Verification items for the finished model (mm, model axes). A direction names the side the tool comes from. Coordinates: 2 decimals unless noted, no trailing zeros. Loops run counter-clockwise (first coordinate to the right, second up) from the corner with the lowest first, then second, coordinate; pieces in that order, holes last. Notation, with made-up numbers: (-19, -22.5) - (-11, -22.5) arc R17 ccw to (-11, -7.5) - close; hole circle Ø7 at (-29.75, 40). An arc over 180 degrees is marked (long way). One line per item, written item: value. Start each with the question number.
(1) Section check A-A (y = 0). Record the boundary of the cut face in (x, z).
(2) Thickness scan on probe 1 along X at (y, z) = (101, -55); probe 2 along X at (y, z) = (-50, 64); probe 3 along Z at (x, y) = (117, -12). Record the ranges inside material, lowest first. Write a range as [from, to].
(3) Section check C-C (x = -96). Record the boundary of the cut face in (y, z).
(4) Section check B-B (z = -59). Count the separate pieces of the cut face and the enclosed holes in it, plus the area to 3 significant figures.
(5) Set-up check for faces 1 (the face through (-35.487, 74.751, 18.458)), 2 (the face through (-153.15, 71.8, -13.56)), 3 (the face through (-75, 99, 1)), 4 (the face through (62.59, 99.15, 59.84)): record each of +Z, -Z, +X, -X, +Y, -Y from which the full face is reachable in a straight line by a thin tool's end or side.
(6) Gauge pin test, flat ends, axial feed: P1, Ø16, axis at x = -55, z = 55, coming from the -Y side; P2, Ø1, axis at x = -121, y = 8, coming from the -Z side; P3, Ø6.5, axis at x = 25.5, y = 103, coming from the +Z side; P4, Ø23.5, axis at y = -20.71, z = 77.27, coming from the -X side. Record the tip position at first contact, or that the pin passes through.
(7) Draft check along X on faces 5 (the face through (-69.297, 99.154, -68.986)), 6 (the face through (-142, 43, -43)), 7 (the face through (153.15, 56.96, 65.56)). Enter one of: +X half, -X half, draft (parallel to the pull), parting line (faces both ways), or undercut.
```python
from build123d import *

# Parameters (mm, degrees)
SKETCH2_R           = 40
SKETCH2_R_2         = 9
BOSS_EXTRUDE1_DEPTH = 22
BOSS_EXTRUDE6_REACH = 286.598
SKETCH2_8_R         = 40
SKETCH2_8_R_2       = 27.5
SKETCH2_8_R_3       = 24
CUT_EXTRUDE5_REACH  = 362.117
SKETCH8_R           = 9


with BuildPart() as part:
    # Sketch1 → Revolve1 (revolve)
    with BuildSketch(Plane.XY, mode=Mode.PRIVATE) as revolve1_sk:
        Polygon((-164, -37.5), (-164, -100), (-142, -100), (-142, -54.482048161), (0, -66.905438381), (142, -54.482048161), (142, -100), (164, -100), (164, -37.5), (0, -51.848140818), align=None)
    revolve(revolve1_sk.sketch.rotate(Axis((0, 0, 0), (-1, 0, 0)), 270), axis=Axis((0, 0, 0), (-1, 0, 0)))

    # Sketch2<8> → Boss-Extrude6 (add, up to next)
    with BuildSketch(Plane(origin=(0, 110, 0), x_dir=(1, 0, 0), z_dir=(0, 1, 0)), mode=Mode.PRIVATE) as boss_extrude6_sk1:
        with Locations(Location((0, 0, 0), (0, 0, 270))):
            Circle(SKETCH2_8_R)
        Circle(SKETCH2_8_R_2, mode=Mode.SUBTRACT)
    boss_extrude6_tool1 = extrude(boss_extrude6_sk1.sketch, amount=-BOSS_EXTRUDE6_REACH, mode=Mode.PRIVATE) - part.part
    # Sketch2<8> → Boss-Extrude6 (add, up to next)
    with BuildSketch(Plane(origin=(0, 110, 0), x_dir=(1, 0, 0), z_dir=(0, 1, 0)), mode=Mode.PRIVATE) as boss_extrude6_sk2:
        Circle(SKETCH2_8_R_2)
        Circle(SKETCH2_8_R_3, mode=Mode.SUBTRACT)
    boss_extrude6_tool2 = extrude(boss_extrude6_sk2.sketch, amount=-BOSS_EXTRUDE6_REACH, mode=Mode.PRIVATE) - part.part
    # Sketch2<8> → Boss-Extrude6 (add, up to next)
    with BuildSketch(Plane(origin=(0, 110, 0), x_dir=(1, 0, 0), z_dir=(0, 1, 0)), mode=Mode.PRIVATE) as boss_extrude6_sk3:
        Circle(SKETCH2_8_R_3)
    boss_extrude6_tool3 = extrude(boss_extrude6_sk3.sketch, amount=-BOSS_EXTRUDE6_REACH, mode=Mode.PRIVATE) - part.part


with BuildPart() as body_2:
    # Sketch2 → Boss-Extrude1 (new body)
    with BuildSketch(Plane(origin=(0, 110, 0), x_dir=(1, 0, 0), z_dir=(0, 1, 0))):
        with BuildLine():
            Line((-55, 75), (55, 75))
            ThreePointArc((55, 75), (69.142135624, 69.142135624), (75, 55))
            Line((75, 55), (75, -55))
            ThreePointArc((75, -55), (69.142135624, -69.142135624), (55, -75))
            Line((55, -75), (-55, -75))
            ThreePointArc((-55, -75), (-69.142135624, -69.142135624), (-75, -55))
            Line((-75, -55), (-75, 55))
            ThreePointArc((-75, 55), (-69.142135624, 69.142135624), (-55, 75))
        make_face()
        with Locations(Location((0, 0, 0), (0, 0, 270))):
            Circle(SKETCH2_R, mode=Mode.SUBTRACT)
        with Locations(Location((55, -55, 0), (0, 0, 270))):
            Circle(SKETCH2_R_2, mode=Mode.SUBTRACT)
        with Locations(Location((-55, -55, 0), (0, 0, 270))):
            Circle(SKETCH2_R_2, mode=Mode.SUBTRACT)
        with Locations(Location((55, 55, 0), (0, 0, 270))):
            Circle(SKETCH2_R_2, mode=Mode.SUBTRACT)
        with Locations(Location((-55, 55, 0), (0, 0, 270))):
            Circle(SKETCH2_R_2, mode=Mode.SUBTRACT)
    extrude(amount=-BOSS_EXTRUDE1_DEPTH)


with BuildPart() as part_1:
    add(part.part)

    add(body_2.part)  # Boss-Extrude6 merges body 2
    add(boss_extrude6_tool1.solids().sort_by_distance((0, 110, -38.868629))[0])
    add(boss_extrude6_tool2.solids().sort_by_distance((-26.722183, 110, 0))[0])
    add(boss_extrude6_tool3.solids().sort_by_distance((0, 110, 0))[0])

    # Sketch7 → Cut-Revolve1 (revolve, cut)
    with BuildSketch(Plane.XY, mode=Mode.PRIVATE) as cut_revolve1_sk:
        Polygon((0, 19.40041476), (0, 110), (27.5, 110), (27.5, 95), (24, 95), (22.680404331, 19.40041476), align=None)
    revolve(cut_revolve1_sk.sketch.rotate(Axis((0, 0, 0), (0, -1, 0)), 180), axis=Axis((0, 0, 0), (0, -1, 0)), mode=Mode.SUBTRACT)

    # Sketch8 → Cut-Extrude5 (cut, up to next)
    with BuildSketch(Plane(origin=(164, 0, 0), x_dir=(0, 0, -1), z_dir=(1, 0, 0)), mode=Mode.PRIVATE) as cut_extrude5_sk1:
        with Locations((-77.274066103, -20.705523608)):
            Circle(SKETCH8_R)
    cut_extrude5_tool1 = extrude(cut_extrude5_sk1.sketch, amount=-CUT_EXTRUDE5_REACH, mode=Mode.PRIVATE) & part_1.part
    # Sketch8 → Cut-Extrude5 (cut, up to next)
    with BuildSketch(Plane(origin=(164, 0, 0), x_dir=(0, 0, -1), z_dir=(1, 0, 0)), mode=Mode.PRIVATE) as cut_extrude5_sk2:
        with Locations((-56.568542495, 56.568542495)):
            Circle(SKETCH8_R)
    cut_extrude5_tool2 = extrude(cut_extrude5_sk2.sketch, amount=-CUT_EXTRUDE5_REACH, mode=Mode.PRIVATE) & part_1.part
    # Sketch8 → Cut-Extrude5 (cut, up to next)
    with BuildSketch(Plane(origin=(164, 0, 0), x_dir=(0, 0, -1), z_dir=(1, 0, 0)), mode=Mode.PRIVATE) as cut_extrude5_sk3:
        with Locations((20.705523608, 77.274066103)):
            Circle(SKETCH8_R)
    cut_extrude5_tool3 = extrude(cut_extrude5_sk3.sketch, amount=-CUT_EXTRUDE5_REACH, mode=Mode.PRIVATE) & part_1.part
    # Sketch8 → Cut-Extrude5 (cut, up to next)
    with BuildSketch(Plane(origin=(164, 0, 0), x_dir=(0, 0, -1), z_dir=(1, 0, 0)), mode=Mode.PRIVATE) as cut_extrude5_sk4:
        with Locations((77.274066103, 20.705523608)):
            Circle(SKETCH8_R)
    cut_extrude5_tool4 = extrude(cut_extrude5_sk4.sketch, amount=-CUT_EXTRUDE5_REACH, mode=Mode.PRIVATE) & part_1.part
    # Sketch8 → Cut-Extrude5 (cut, up to next)
    with BuildSketch(Plane(origin=(164, 0, 0), x_dir=(0, 0, -1), z_dir=(1, 0, 0)), mode=Mode.PRIVATE) as cut_extrude5_sk5:
        with Locations((56.568542495, -56.568542495)):
            Circle(SKETCH8_R)
    cut_extrude5_tool5 = extrude(cut_extrude5_sk5.sketch, amount=-CUT_EXTRUDE5_REACH, mode=Mode.PRIVATE) & part_1.part
    # Sketch8 → Cut-Extrude5 (cut, up to next)
    with BuildSketch(Plane(origin=(164, 0, 0), x_dir=(0, 0, -1), z_dir=(1, 0, 0)), mode=Mode.PRIVATE) as cut_extrude5_sk6:
        with Locations((-20.705523608, -77.274066103)):
            Circle(SKETCH8_R)
    cut_extrude5_tool6 = extrude(cut_extrude5_sk6.sketch, amount=-CUT_EXTRUDE5_REACH, mode=Mode.PRIVATE) & part_1.part
    cut_extrude5_1 = cut_extrude5_tool1.solids().sort_by_distance((164, -20.705524, 77.274066))[0]
    add(cut_extrude5_1, mode=Mode.SUBTRACT)
    cut_extrude5_2 = cut_extrude5_tool2.solids().sort_by_distance((164, 56.568542, 56.568542))[0]
    add(cut_extrude5_2, mode=Mode.SUBTRACT)
    cut_extrude5_3 = cut_extrude5_tool3.solids().sort_by_distance((164, 77.274066, -20.705524))[0]
    add(cut_extrude5_3, mode=Mode.SUBTRACT)
    cut_extrude5_4 = cut_extrude5_tool4.solids().sort_by_distance((164, 20.705524, -77.274066))[0]
    add(cut_extrude5_4, mode=Mode.SUBTRACT)
    cut_extrude5_5 = cut_extrude5_tool5.solids().sort_by_distance((164, -56.568542, -56.568542))[0]
    add(cut_extrude5_5, mode=Mode.SUBTRACT)
    cut_extrude5_6 = cut_extrude5_tool6.solids().sort_by_distance((164, -77.274066, 20.705524))[0]
    add(cut_extrude5_6, mode=Mode.SUBTRACT)
    cut_extrude5 = cut_extrude5_1 + cut_extrude5_2 + cut_extrude5_3 + cut_extrude5_4 + cut_extrude5_5 + cut_extrude5_6  # Cut-Extrude5 as one shape, for the pattern or mirror that repeats it

    # Mirror1: Cut-Extrude5 across plane
    add(cut_extrude5.mirror(Plane(origin=(0, 0, 0), x_dir=(0, 0, 1), z_dir=(1, 0, 0))), mode=Mode.SUBTRACT)


solid = part_1.part
```
Responses:
1. outline: (-164, -100) - (-142, -100) - (-142, -54.48) - (0, -66.91) - (142, -54.48) - (142, -100) - (164, -100) - (164, -37.5) - (0, -51.85) - (-164, -37.5) - close; (-164, 37.5) - (0, 51.85) - (164, 37.5) - (164, 100) - (142, 100) - (142, 54.48) - (0, 66.91) - (-142, 54.48) - (-142, 100) - (-164, 100) - close
2. probe 1: x = [-75, -64], [-46, 46], [64, 75]
2. probe 2: x = [-164, -142], [142, 164]
2. probe 3: z = [-55.38, -39.84], [39.84, 55.38]
3. outline: circle Ø117.01 at (0, 0); hole circle Ø86.9 at (0, 0)
4. separate pieces: 8
4. enclosed holes: 0
4. area: 16,400 mm²
5. face 1: none
5. face 2: -X
5. face 3: +Z, -Z, +Y
5. face 4: +Y
6. P1: stops at y = -40.64
6. P2: stops at z = -55.83
6. P3: stops at z = 75
6. P4: stops at x = -164
7. face 5: -X half
7. face 6: undercut
7. face 7: draft
